Here's the drawing with two shaded views (mm, measured from the low corner). I have some questions. Coordinates: 2 decimals unless noted, no trailing zeros. Order: outer loops, then holes, each group sorted by start corner. A loop starts at its lowest first (then second) coordinate and runs counter-clockwise, first axis right, second up. Notation, with made-up numbers: (22, 54) -> (49, 54) arc R24 cw to (49, 70) -> close; hole circle Ø3 at (23.25, 12.5). An arc over 180 degrees is marked (long way). One line per item, written item: value. Start each with the question number.
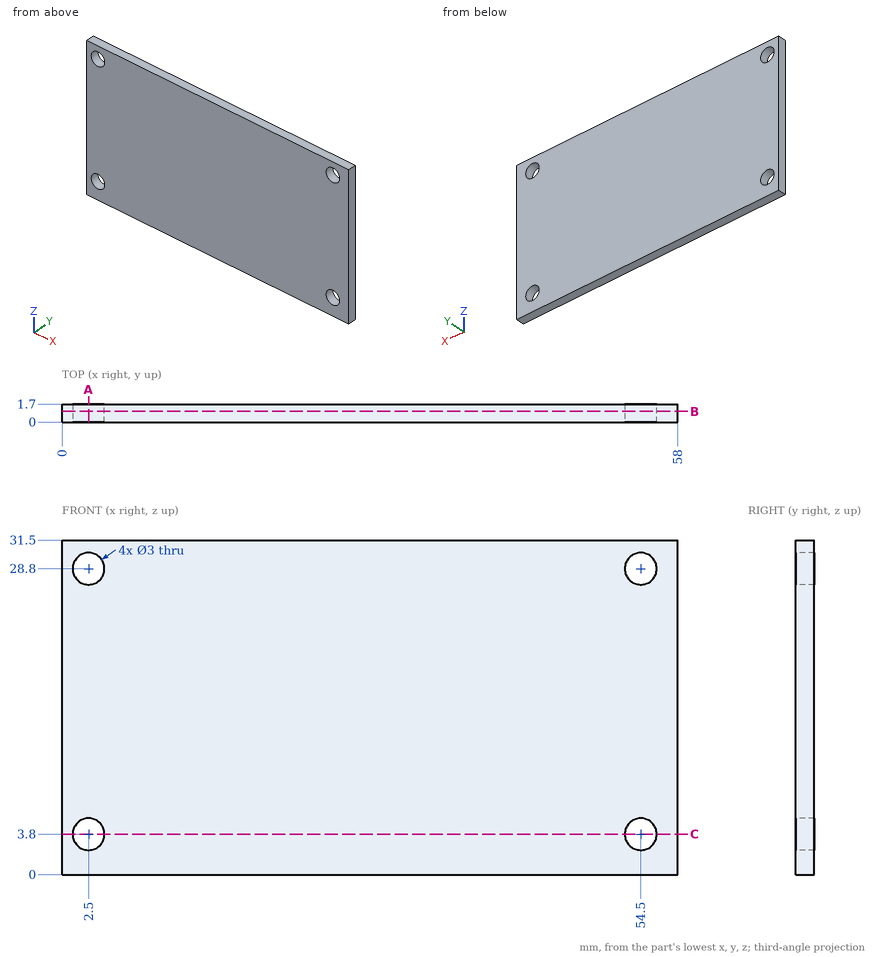
Q1. Imagine slicing it at C-C (z = 3.8). Write out the boundary of the cut face in (x, y).
Q2. For P1, Ø2.5, axis at x = 2.5, z = 28.8, coming from the +Y side, with a flat end and sliding along its axis, tell me the tip position at first contact or that it passes through.
Q3. I need wall thicknesses on line 1 (Z direction, x = 54.5, y = 1.3); line 2 (X direction, y = 1.1, z = 29.5); line 3 (X direction, y = 1.1, z = 5). Which ranges of each line are inside material? Lowest first, please.
Q4. Imagine slicing it at B-B (y = 1). Write out the boundary of the cut face in (x, z), plus the area to 3 significant figures.
Q5. Imagine slicing it at A-A (x = 2.5). Write out the boundary of the cut face in (y, z).
Completed:
1. outline: (0, 0) -> (1, 0) -> (1, 1.7) -> (0, 1.7) -> close; (4, 0) -> (53, 0) -> (53, 1.7) -> (4, 1.7) -> close; (56, 0) -> (58, 0) -> (58, 1.7) -> (56, 1.7) -> close
2. P1: passes through
3. line 1: z = 0 to 2.3, 5.3 to 27.3, 30.3 to 31.5
3. line 2: x = 0 to 1.17, 3.83 to 53.17, 55.83 to 58
3. line 3: x = 0 to 1.6, 3.4 to 53.6, 55.4 to 58
4. outline: (0, 0) -> (58, 0) -> (58, 31.5) -> (0, 31.5) -> close; hole circle Ø3 at (2.5, 3.8); hole circle Ø3 at (2.5, 28.8); hole circle Ø3 at (54.5, 3.8); hole circle Ø3 at (54.5, 28.8)
4. area: 1,800 mm2
5. outline: (0, 0) -> (1.7, 0) -> (1.7, 2.3) -> (0, 2.3) -> close; (0, 5.3) -> (1.7, 5.3) -> (1.7, 27.3) -> (0, 27.3) -> close; (0, 30.3) -> (1.7, 30.3) -> (1.7, 31.5) -> (0, 31.5) -> close
